Can you work these out from the drawing? Everything is in mm from the part's minimum corner. Round coordinates to 2 decimals unless told otherwise and drop trailing zeros. Loops run counter-clockwise (first coordinate to the right, second up) from the corner with the lowest first, then second, coordinate; pieces in that order, holes last. Notation, with made-up numbers: (51, 15.5) -> (70, 15.5) arc R27 ccw to (70, 38.5) -> close; hole circle Ø1 at (-23, 65.5). An arc over 180 degrees is marked (long way). One line per item, written item: value.
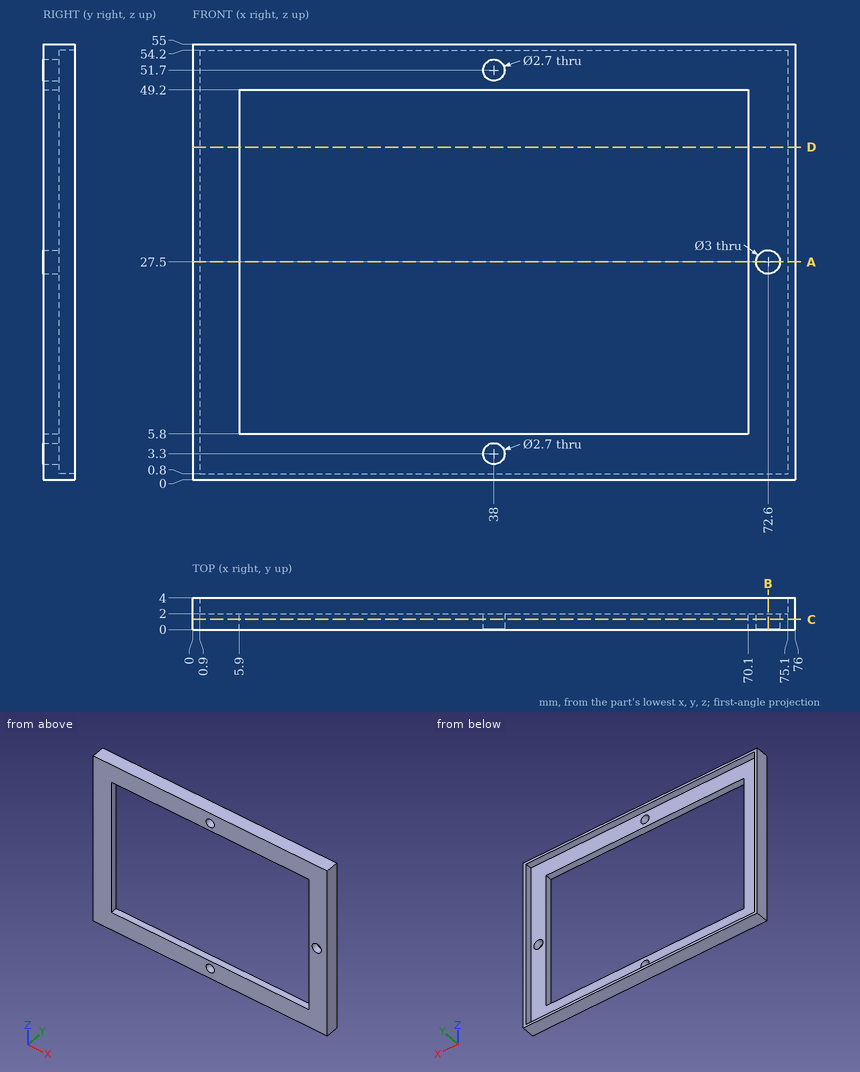
(1) Please list where these lines run through material, in increasing order: L1, parallel to Z at x = 38, y = 0.7; L2, parallel to X at y = 1.3, z = 27.5; L3, parallel to Z at x = 41, y = 3.05.
Results below:
L1: z = 0 to 1.95, 4.65 to 5.8, 49.2 to 50.35, 53.05 to 55
L2: x = 0 to 5.9, 70.1 to 71.1, 74.1 to 76
L3: z = 0 to 0.8, 54.2 to 55
(2) Imagine slicing it at C-C on y = 1.3. Write out the boundary of the cut face in (x, z).
Results below:
outline: (0, 0) -> (76, 0) -> (76, 55) -> (0, 55) -> close; hole (5.9, 5.8) -> (70.1, 5.8) -> (70.1, 49.2) -> (5.9, 49.2) -> close; hole circle Ø2.7 at (38, 3.3); hole circle Ø2.7 at (38, 51.7); hole circle Ø3 at (72.6, 27.5)
(3) Imagine slicing it at A-A on z = 27.5. Write out the boundary of the cut face in (x, y), then the cut area to 3 significant figures.
Results below:
outline: (0, 0) -> (5.9, 0) -> (5.9, 2) -> (0.9, 2) -> (0.9, 4) -> (0, 4) -> close; (70.1, 0) -> (71.1, 0) -> (71.1, 2) -> (70.1, 2) -> close; (74.1, 0) -> (76, 0) -> (76, 4) -> (75.1, 4) -> (75.1, 2) -> (74.1, 2) -> close
area: 21.2 mm²
(4) Imagine slicing it at D-D on z = 42. Write out the boundary of the cut face in (x, y).
Results below:
outline: (0, 0) -> (5.9, 0) -> (5.9, 2) -> (0.9, 2) -> (0.9, 4) -> (0, 4) -> close; (70.1, 0) -> (76, 0) -> (76, 4) -> (75.1, 4) -> (75.1, 2) -> (70.1, 2) -> close
(5) For pin 1 Ø1.6 at (x, z) = (38, 51.7) entering from -Y (1 decimal); pin 2 Ø0.6 at (y, z) = (3, 40) entering from -X; pin 3 Ø10 at (x, z) = (57, 7.5) entering from +Y, each with a flat end and sliding along its axis, tell me the tip position at first contact or that it passes through.
Results below:
pin 1: passes through
pin 2: stops at x = 0
pin 3: stops at y = 2
(6) Imagine slicing it at B-B on x = 72.6. Write out the boundary of the cut face in (y, z), then the cut area to 3 significant figures.
Results below:
outline: (0, 0) -> (4, 0) -> (4, 0.8) -> (2, 0.8) -> (2, 26) -> (0, 26) -> close; (0, 29) -> (2, 29) -> (2, 54.2) -> (4, 54.2) -> (4, 55) -> (0, 55) -> close
area: 107 mm²
